Build history of the part. All positions in model axes, mm. A direction names the side the tool comes from. Give positions to 0.01 mm unless a question says otherwise; leave off trailing zeros. Write each loop counter-clockwise with the first axis right and the second up, starting at its lowest first coordinate (ties: lowest second). Pieces come first, ordered by that corner, then holes. Notation, with made-up numbers: (52, 22) -> (99, 22) arc R31 ccw to (99, 48) -> close; hole circle Ø3 at (87.5, 74). An arc over 180 degrees is marked (long way). Write item = value, one per line. Start each with the question number.
Q1. Saw through at D-D, the plane x = 5.5. List the corners of the cut face in (y, z), then the cut area to 3 significant figures.
Q2. Wall check: line 1 (X direction, y = 1, z = 9.5); line 2 (Y direction, x = -5, z = 1.5); line 3 (X direction, y = 3, z = 6.75). Give the ranges that are in metal, low to high.
Q3. Mould opens along Y. For faces 1 (the face through (-1.66, 7.5, 4.93)), 2 (the face through (-0.16, -7.4, 4.93)), 3 (the face through (1, 4, 10)) say: pulls with the +Y half, pulls with the -Y half, needs draft (parallel to the pull), parting line crosses it, or undercut.
Q4. Saw through at A-A, the plane x = 3.5. List the corners of the cut face in (y, z).
Q5. Saw through at B-B, the plane y = 4. List the corners of the cut face in (x, z), then the cut area to 3 significant figures.
Q6. Drop flat-ended pins along their axis: P1, Ø3, axis at x = 5, z = 6, coming from the +Y side; P2, Ø1.5, axis at x = 4.5, y = 3, coming from the +Z side; P3, Ø1.5, axis at y = -1.5, z = 1, coming from the +X side; P4, Ø5, axis at x = -5.5, z = 5, coming from the -Y side. Give the stop position or say it passes through.
Q7. Saw through at C-C, the plane z = 8. List the corners of the cut face in (x, y).
Q8. Tool access for faces 4 (the face through (0, -6, 5)), 5 (the face through (-1.304, 8.898, 4.93)), 6 (the face through (-10, 0, 5)): list every direction of +Z, -Z, +X, -X, +Y, -Y with a clear straight run to the whole face (end or side of a thin tool).
from build123d import *

# Parameters (mm, degrees)
F1_DEPTH = 10


with BuildPart() as f1:
    # F0 (on Top) → F1 (new body)
    with BuildSketch(Plane.XY):
        with BuildLine():
            ThreePointArc((0, 4.242641), (2.174235, 2.598076), (3, 0))
            Line((3, 0), (4.4, 0))
            ThreePointArc((4.4, 0), (3.31733, 3.406367), (0.466667, 5.562573))
            ThreePointArc((0.466667, 5.562573), (-4.906367, 4.81733), (-7.4, 0))
            ThreePointArc((-7.4, 0), (0, -7.4), (7.4, 0))
            ThreePointArc((7.4, 0), (-1.5, 8.9), (-10.4, 0))
            Line((-10.4, 0), (-9, 0))
            ThreePointArc((-9, 0), (-1.5, 7.5), (6, 0))
            ThreePointArc((6, 0), (0, -6), (-6, 0))
            ThreePointArc((-6, 0), (-4.098076, 3.674235), (0, 4.242641))
        make_face()
    extrude(amount=F1_DEPTH)


solid = f1.part
Report:
q1.outline = (-4.95, 0) -> (-2.4, 0) -> (-2.4, 10) -> (-4.95, 10) -> close; (2.69, 0) -> (5.5, 0) -> (5.5, 10) -> (2.69, 10) -> close
q1.area = 53.6 mm2
q2.line_1 = -10.34 to -8.93, -7.31 to -5.89, 2.89 to 4.31, 5.93 to 7.34
q2.line_2 = -5.46 to -3.32, 2.83 to 4.75, 6.63 to 8.18
q2.line_3 = -9.88 to -8.37, -6.58 to -4.85, 1.85 to 3.58, 5.37 to 6.88
q3.face_1 = undercut
q3.face_2 = pulls with the -Y half
q3.face_3 = needs draft
q4.outline = (-6.52, 0) -> (-4.87, 0) -> (-4.87, 10) -> (-6.52, 10) -> close; (0, 0) -> (3.13, 0) -> (3.13, 10) -> (0, 10) -> close; (5.59, 0) -> (7.36, 0) -> (7.36, 10) -> (5.59, 10) -> close
q5.outline = (-9.45, 0) -> (-7.84, 0) -> (-7.84, 10) -> (-9.45, 10) -> close; (-5.84, 0) -> (-3.56, 0) -> (-3.56, 10) -> (-5.84, 10) -> close; (0.56, 0) -> (2.84, 0) -> (2.84, 10) -> (0.56, 10) -> close; (4.84, 0) -> (6.45, 0) -> (6.45, 10) -> (4.84, 10) -> close
q5.area = 77.6 mm2
q6.P1 = 7.36
q6.P2 = through
q6.P3 = 7.36
q6.P4 = -6.76
q7.outline = (-10.4, 0) -> (-9, 0) arc R7.5 cw to (6, 0) arc R6 cw to (-6, 0) arc R4.5 cw to (3, 0) -> (4.4, 0) arc R5.9 ccw to (0.47, 5.56) arc R5.9 ccw to (-7.4, 0) arc R7.4 ccw to (7.4, 0) arc R8.9 ccw to start
q8.face_4 = +Z, -Z
q8.face_5 = +Z, -Z, +Y
q8.face_6 = +Z, -Z, -X, -Y
